Work out the finished part from the listing and answer in its coordinate system (mm). A direction names the side the tool comes from. Coordinates: 2 decimals unless noted, no trailing zeros. Loops run counter-clockwise (first coordinate to the right, second up) from the corner with the lowest first, then second, coordinate; pieces in that order, holes last. Notation, with made-up numbers: (-5, 41) -> (35, 41) arc R23 ccw to (35, 78) -> close; hole circle Ø6 at (40, 43). An arc over 180 degrees is marked (long way). Use a Markdown table: item, result.
from build123d import *

# Parameters (mm, degrees)
F1_DEPTH = 2.5
F2_R     = 1.5
F3_DEPTH = 1
F4_R     = 0.49999


# Not quite as in the source:
# - a fillet or chamfer is up to 0.001 mm smaller than in the source, because OpenCascade refuses the exact size


with BuildPart() as f1:
    # F0 (on Right) → F1 (new body, symmetric)
    with BuildSketch(Plane.YZ):
        Polygon((-7.5, 0), (7.5, 0), (7.5, 1), (-6.5, 1), (-6.5, 20), (-7.5, 20), align=None)
    extrude(amount=F1_DEPTH, both=True)

    # F2 (on face) → F3 (cut, through all)
    with BuildSketch(Plane.XY.offset(1)):
        with Locations((0, 3.5)):
            Circle(F2_R)
        with Locations((0, -3.5)):
            Circle(F2_R)
    extrude(amount=-F3_DEPTH, mode=Mode.SUBTRACT)

    # F4 (radius 0.5 in the source; OpenCascade refuses exactly that, so slightly less here)
    f4_edges = [f1.edges().sort_by_distance(p)[0] for p in [
        (0, -6.5, 20),
        (0, -7.5, 20),
    ]]
    fillet(f4_edges, radius=F4_R)


solid = f1.part
Q1. Section B-B on y = 3.5 is taken. Determine the outline of the cut face in (x, z).
Solved:
| item | result |
|---|---|
| outline | (-2.5, 0) -> (-1.5, 0) -> (-1.5, 1) -> (-2.5, 1) -> close; (1.5, 0) -> (2.5, 0) -> (2.5, 1) -> (1.5, 1) -> close |
Q2. Determine the mould class of faces 3 (the flat face through (-2.5, -7, 7)), 4 (the flat face through (0, -6.5, 10)), 5 (the cylindrical face through (-0.195, -2.013, 0.507)), 6 (the flat face through (2.5, -7, 7)) for opening direction X: pulls with the +X half, pulls with the -X half, needs draft (parallel to the pull), parting line crosses it, or undercut.
Solved:
| item | result |
|---|---|
| face 3 | pulls with the -X half |
| face 4 | needs draft |
| face 5 | undercut |
| face 6 | pulls with the +X half |
Q3. Section A-A on x = 0.9 is taken. State how many separate pieces and enclosed holes the cut face has, and give its area (3 significant figures).
Solved:
| item | result |
|---|---|
| separate pieces | 3 |
| enclosed holes | 0 |
| area | 29.1 mm² |
Q4. Given pin 1 Ø2.5 at (x, y) = (0, -3.5) entering from +Z; pin 2 Ø6 at (y, z) = (-4, 16) entering from -X; pin 3 Ø3 at (x, z) = (1.5, 7.5) entering from +Y; pin 4 Ø1.5 at (x, y) = (-1.5, -4) entering from +Z, each flat-ended and moving along its own axis, determine where each tip first touches the part or whether it passes through.
Solved:
| item | result |
|---|---|
| pin 1 | through |
| pin 2 | x = -2.5 |
| pin 3 | y = -6.5 |
| pin 4 | z = 1 |
Q5. For faces 1 (the flat face through (0, -7.5, 10)), 2 (the flat face through (0, 1, 1)), determine the directions among +Z, -Z, +X, -X, +Y, -Y from which every point of the face is accessible in a straight line to the end or side of a thin tool.
Solved:
| item | result |
|---|---|
| face 1 | +Z, -Z, +X, -X, -Y |
| face 2 | +Z, +X, -X, +Y |
Q6. Consider line 1 (Y direction, x = 0, z = 0.6); line 2 (Z direction, x = 0.9, y = 1); line 3 (Y direction, x = -1.35, z = 7.5). Determine where each line is inside the solid, lowest interval first. Write a range as [from, to].
Solved:
| item | result |
|---|---|
| line 1 | [-7.5, -5], [-2, 2], [5, 7.5] |
| line 2 | [0, 1] |
| line 3 | [-7.5, -6.5] |
